```python
from build123d import *

# Parameters (mm, degrees)
EXTRUDE_THIN1_DEPTH = 2.5


with BuildPart() as part:
    # Sketch1 → Extrude-Thin1 (new body, symmetric)
    with BuildSketch(Plane.XY):
        with BuildLine():
            Line((-248, -24.5), (-33, -24.5))
            ThreePointArc((-33, -24.5), (-27.56956187, -23.194850479), (-23.325321853, -19.564492338))
            Line((-23.325321853, -19.564492338), (-5.991014082, 4.343702368))
            ThreePointArc((-5.991014082, 4.343702368), (0, 7.4), (5.991014082, 4.343702368))
            Line((5.991014082, 4.343702368), (23.325321853, -19.564492338))
            ThreePointArc((23.325321853, -19.564492338), (27.56956187, -23.194850479), (33, -24.5))
            Line((33, -24.5), (248, -24.5))
            Line((248, -24.5), (248, -25.8))
            Line((248, -25.8), (33, -25.8))
            ThreePointArc((33, -25.8), (26.978802911, -24.352867686), (22.272846406, -20.327575186))
            Line((22.272846406, -20.327575186), (4.938538636, 3.58061952))
            ThreePointArc((4.938538636, 3.58061952), (0, 6.1), (-4.938538636, 3.58061952))
            Line((-4.938538636, 3.58061952), (-22.272846406, -20.327575186))
            ThreePointArc((-22.272846406, -20.327575186), (-26.978802911, -24.352867686), (-33, -25.8))
            Line((-33, -25.8), (-248, -25.8))
            Line((-248, -25.8), (-248, -24.5))
        make_face()
    extrude(amount=EXTRUDE_THIN1_DEPTH, both=True)


solid = part.part
```
For this review, take the finished solid that the model builds, in its own axes (mm). Round coordinates to 2 decimals unless told otherwise and drop trailing zeros. Write each loop counter-clockwise with the first axis right and the second up, starting at its lowest first coordinate (ties: lowest second). Pieces come first, ordered by that corner, then holes. Notation, with made-up numbers: (83, 45.25) -> (127, 45.25) arc R13 cw to (127, 62.25) -> close; hole circle Ø5 at (64.25, 33.5). An arc over 180 degrees is marked (long way). One line per question, with ' | ' between items. Start each with the question number.
1) Wall thickness on line 1 along Y through (x, z) = (158, 0.15); line 2 along X through (y, z) = (-4, 1.4); line 3 along X through (y, z) = (1, -1.7): over which ranges is each line inside the solid? List them lowest first.
2) Add section B-B (y = -11.5). Write out the cut boundary in (x, z), and give its area (3 significant figures).
3) Mouldability with a two-part tool opening along X and no side actions: class faces 1 (the flat face through (-13.484, -8.206, 0.035)), 2 (the flat face through (13.727, -8.541, 0.035)), 3 (the flat face through (14.537, -7.443, 0.035)), 4 (the flat face through (-14.78, -7.78, 0.04)) as +X half, -X half, draft (parallel to the pull), parting line (faces both ways), or undercut.
4) Add section C-C (x = -76). Write out the cut boundary in (y, z).
5) Add section A-A (z = 0.85). Write out the cut boundary in (x, y).
6) For pin 1 Ø12 at (x, y) = (-179.5, -17.5) entering from -Z; pin 2 Ø3 at (y, z) = (-20.5, 1) entering from -X, all flat-tipped, find the tip position at first contact; note any pin that passes through.
Reported:
1) line 1: y = -25.8 to -24.5 | line 2: x = -12.04 to -10.43, 10.43 to 12.04 | line 3: x = -8.42 to -6.81, 6.81 to 8.42
2) outline: (-17.48, -2.5) -> (-15.87, -2.5) -> (-15.87, 2.5) -> (-17.48, 2.5) -> close; (15.87, -2.5) -> (17.48, -2.5) -> (17.48, 2.5) -> (15.87, 2.5) -> close | area: 16.1 mm²
3) face 1: undercut | face 2: undercut | face 3: +X half | face 4: -X half
4) outline: (-25.8, -2.5) -> (-24.5, -2.5) -> (-24.5, 2.5) -> (-25.8, 2.5) -> close
5) outline: (-248, -25.8) -> (-33, -25.8) arc R13.25 ccw to (-22.27, -20.33) -> (-4.94, 3.58) arc R6.1 cw to (4.94, 3.58) -> (22.27, -20.33) arc R13.25 ccw to (33, -25.8) -> (248, -25.8) -> (248, -24.5) -> (33, -24.5) arc R11.95 cw to (23.33, -19.56) -> (5.99, 4.34) arc R7.4 ccw to (-5.99, 4.34) -> (-23.33, -19.56) arc R11.95 cw to (-33, -24.5) -> (-248, -24.5) -> close
6) pin 1: passes through | pin 2: stops at x = -25.69
